Build history of the part. All positions in model axes, mm. Face numbers are marked on the shaded views. A direction names the side the tool comes from. Round coordinates to 2 decimals unless told otherwise and drop trailing zeros. Order: outer loops, then holes, each group sorted by start corner. A loop starts at its lowest first (then second) coordinate and runs counter-clockwise, first axis right, second up. Notation, with made-up numbers: (-13, 64) -> (4, 64) arc R23 cw to (4, 89) -> close; hole circle Ø5 at (56.5, 63). An arc over 180 degrees is marked (long way). Use a Markdown table: item, result. Add a question column.
Item 1: 3-axis set-ups, long thin cutter, end or side, ignore diameter. For the marked faces 1 and 2: which of +Z, -Z, +X, -X, +Y, -Y reach the whole face in a straight line?
Item 2: Pin check, flat tips, straight feed: pin 1 (4 mm diameter, centred on x = 6.5, y = -3.5, fed in from -Z); pin 2 (10 mm diameter, centred on y = -8, z = 13.5, fed in from -X); pin 3 (8 mm diameter, centred on y = -7.5, z = 12, fed in from -X). Stop position of each tip, or through.
Item 3: Probe L1, parallel to Z at x = -8.25, y = -7; L2, parallel to X at y = 0.5, z = 16.5; L3, parallel to Y at x = 1, z = 1. List the from-to ranges inside material, lowest first.
Item 4: Slice it at B-B, the plane y = 8. Give the cut face in (x, z).
Item 5: Slice it at D-D, the plane z = 0.5. Give the cut face in (x, y).
Item 6: Slice it at C-C, the plane x = 9.5. Give the cut face in (y, z), plus the area to 3 significant figures.
Item 7: Slice it at A-A, the plane z = 33.5. Give the cut face in (x, y).
Item 8: Two-plate mould, pull along X, no slides. Class the marked faces 3, 4 and 5: released by +X, released by -X, zero draft, split by the parting line, or undercut.
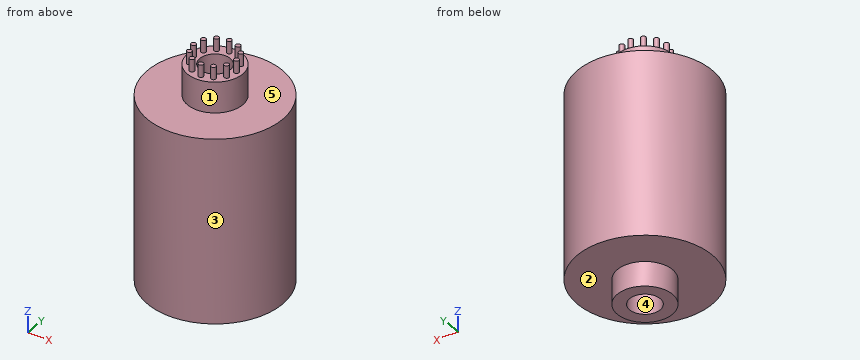
from build123d import *

# Parameters (mm, degrees)
SKETCH2_R           = 11
BOSS_EXTRUDE1_DEPTH = 30
SKETCH3_R           = 4.5
BOSS_EXTRUDE2_DEPTH = 5
BOSS_EXTRUDE3_START = 4
SKETCH4_R           = 4.5
BOSS_EXTRUDE3_DEPTH = 4
SKETCH5_R           = 2.5
CUT_EXTRUDE1_DEPTH  = 42.98809355
SKETCH6_R           = 0.4
BOSS_EXTRUDE4_DEPTH = 2
CIRPATTERN1_COUNT   = 12


with BuildPart() as part:
    # Sketch2 → Boss-Extrude1 (new body)
    with BuildSketch(Plane.XY):
        Circle(SKETCH2_R)
    extrude(amount=BOSS_EXTRUDE1_DEPTH)

    # Sketch3 → Boss-Extrude2 (add)
    with BuildSketch(Plane.XY.offset(30)):
        Circle(SKETCH3_R)
    extrude(amount=BOSS_EXTRUDE2_DEPTH)

    # Sketch4 → Boss-Extrude3 (add)
    with BuildSketch(Plane(origin=(0, 0, 0), x_dir=(-1, 0, 0), z_dir=(0, 0, -1)).offset(BOSS_EXTRUDE3_START)):
        with Locations(Location((0, 0, 0), (0, 0, 180))):
            Circle(SKETCH4_R)
    extrude(amount=-BOSS_EXTRUDE3_DEPTH)

    # Sketch5 → Cut-Extrude1 (cut, through all)
    with BuildSketch(Plane.XY.offset(35)):
        Circle(SKETCH5_R)
    extrude(amount=-CUT_EXTRUDE1_DEPTH, mode=Mode.SUBTRACT)

    # Sketch6 → Boss-Extrude4 (add)
    with BuildSketch(Plane.XY.offset(35)):
        with Locations((0, 3.5)):
            Circle(SKETCH6_R)
    boss_extrude4 = extrude(amount=BOSS_EXTRUDE4_DEPTH)

    # CirPattern1: Boss-Extrude4 ×12 about axis
    cirpattern1_axis = Axis((0, 0, 0), (0, 0, 1))
    for i in range(1, CIRPATTERN1_COUNT):
        add(boss_extrude4.rotate(cirpattern1_axis, i * 360 / CIRPATTERN1_COUNT))


solid = part.part
Check sheet entries:
| question | item | result |
|---|---|---|
| 1 | face 1 | +Z |
| 1 | face 2 | -Z |
| 2 | pin 1 | z = 0 |
| 2 | pin 2 | x = -10.58 |
| 2 | pin 3 | x = -10.43 |
| 3 | L1 | 0 to 30 |
| 3 | L2 | -10.99 to -2.45, 2.45 to 10.99 |
| 3 | L3 | -10.95 to -2.29, 2.29 to 10.95 |
| 4 | outline | (-7.55, 0) -> (7.55, 0) -> (7.55, 30) -> (-7.55, 30) -> close |
| 5 | outline | circle Ø22 at (0, 0); hole circle Ø5 at (0, 0) |
| 6 | outline | (-5.55, 0) -> (5.55, 0) -> (5.55, 30) -> (-5.55, 30) -> close |
| 6 | area | 333 mm2 |
| 7 | outline | circle Ø9 at (0, 0); hole circle Ø5 at (0, 0) |
| 8 | face 3 | split by the parting line |
| 8 | face 4 | undercut |
| 8 | face 5 | zero draft |
